from build123d import *

# Parameters (mm, degrees)
BACK_PLATE_DEPTH    = 2
SKETCH3_R           = 39.1
SKETCH3_R_2         = 37.1
BOSS_EXTRUDE2_DEPTH = 4


with BuildPart() as part:
    # Sketch2 → Back Plate (new body)
    with BuildSketch(Plane.XY.offset(1.869079413)):
        with BuildLine():
            ThreePointArc((-22.788405672, 36.551599508), (-51.432945039, 29.694824664), (-43.048816559, 1.45953847))
            ThreePointArc((-43.048816559, 1.45953847), (-43.466528344, 1.037157748), (-43.724007211, 0.501813707))
            ThreePointArc((-43.724007211, 0.501813707), (-43.795371043, 0), (-43.724007211, -0.501813707))
            ThreePointArc((-43.724007211, -0.501813707), (-43.466528344, -1.037157748), (-43.048816559, -1.45953847))
            ThreePointArc((-43.048816559, -1.45953847), (-51.432945039, -29.694824664), (-22.788405672, -36.551599508))
            ThreePointArc((-22.788405672, -36.551599508), (-22.63146913, -37.124538886), (-22.296587024, -37.615194147))
            ThreePointArc((-22.296587024, -37.615194147), (-21.897685521, -37.927903891), (-21.427420187, -38.117007854))
            ThreePointArc((-21.427420187, -38.117007854), (-20.835059214, -38.161696634), (-20.260410887, -38.011137978))
            ThreePointArc((-20.260410887, -38.011137978), (0, -59.389649327), (20.260410887, -38.011137978))
            ThreePointArc((20.260410887, -38.011137978), (20.835059214, -38.161696634), (21.427420187, -38.117007854))
            ThreePointArc((21.427420187, -38.117007854), (21.897685521, -37.927903891), (22.296587024, -37.615194147))
            ThreePointArc((22.296587024, -37.615194147), (22.63146913, -37.124538886), (22.788405672, -36.551599508))
            ThreePointArc((22.788405672, -36.551599508), (51.432945039, -29.694824664), (43.048816559, -1.45953847))
            ThreePointArc((43.048816559, -1.45953847), (43.466528344, -1.037157748), (43.724007211, -0.501813707))
            ThreePointArc((43.724007211, -0.501813707), (43.795371043, 0), (43.724007211, 0.501813707))
            ThreePointArc((43.724007211, 0.501813707), (43.466528344, 1.037157748), (43.048816559, 1.45953847))
            ThreePointArc((43.048816559, 1.45953847), (51.432945039, 29.694824664), (22.788405672, 36.551599508))
            ThreePointArc((22.788405672, 36.551599508), (22.63146913, 37.124538886), (22.296587024, 37.615194147))
            ThreePointArc((22.296587024, 37.615194147), (21.897685521, 37.927903891), (21.427420187, 38.117007854))
            ThreePointArc((21.427420187, 38.117007854), (20.835059214, 38.161696634), (20.260410887, 38.011137978))
            ThreePointArc((20.260410887, 38.011137978), (0, 59.389649327), (-20.260410887, 38.011137978))
            ThreePointArc((-20.260410887, 38.011137978), (-21.897685521, 37.927903891), (-22.788405672, 36.551599508))
        make_face()
        with BuildLine():
            Line((-31, 20.381609357), (-31, -20.381609357))
            ThreePointArc((-31, -20.381609357), (0, -37.1), (31, -20.381609357))
            Line((31, -20.381609357), (31, 20.381609357))
            ThreePointArc((31, 20.381609357), (0, 37.1), (-31, 20.381609357))
        make_face(mode=Mode.SUBTRACT)
    extrude(amount=BACK_PLATE_DEPTH)

    # Sketch3 → Boss-Extrude2 (add)
    with BuildSketch(Plane.XY.offset(3.869079413)):
        Circle(SKETCH3_R)
        with Locations(Location((0, 0, 0), (0, 0, 146.676229541))):
            Circle(SKETCH3_R_2, mode=Mode.SUBTRACT)
    extrude(amount=BOSS_EXTRUDE2_DEPTH)


solid = part.part
Design review of the part built by this model. Coordinates are the model's own, in mm. A direction names the side the tool comes from. Round coordinates to 2 decimals unless told otherwise and drop trailing zeros. Write each loop counter-clockwise with the first axis right and the second up, starting at its lowest first coordinate (ties: lowest second). Pieces come first, ordered by that corner, then holes. Notation, with made-up numbers: (30.25, 10.25) - (83.25, 10.25) arc R23 ccw to (83.25, 33.25) - close; hole circle Ø7 at (52.25, -30). An arc over 180 degrees is marked (long way). Use a Markdown table: item, result. Add a question column.
1. For faces 1 (the face through (33, 0, 3.869)), 2 (the face through (14, -35, 7.869)), list the 3-axis set-ups (+Z, -Z, +X, -X, +Y, -Y) from which the entire face can be reached by the end or side of a thin tool; tool diameter is ignored.
2. Mouldability with a two-part tool opening along Y and no side actions: class faces 3 (the face through (51.2, -30.09, 2.86)), 4 (the face through (-37, 1, 1.869)), 5 (the face through (37.294, 11.745, 5.841)) as +Y half, -Y half, draft (parallel to the pull), parting line (faces both ways), or undercut.
3. Clearance check with flat-ended pins moving along their axes: pin 1 (3 mm diameter, centred on y = 27.5, z = 5, fed in from -X); pin 2 (3 mm diameter, centred on x = -8.5, z = 6, fed in from +Y); pin 3 (1.5 mm diameter, centred on x = -40.5, z = 7, fed in from +Y); pin 4 (1.6 mm diameter, centred on y = 8, z = 3, fed in from -X). State where each tip first meets the part, or that it passes through.
4. We need section C-C (z = 5.2). State the section outline as (x, y) points, then the cut area to 3 significant figures.
5. Wall thickness on probe 1 along Y at (x, z) = (0, 4.9); probe 2 along Y at (x, z) = (46.5, 2.4); probe 3 along Z at (x, y) = (22.5, -32.5): over which ranges is each line inside the solid? List them lowest first.
6. We need section D-D (y = 10.5). State the section outline as (x, z) points.
7. We need section A-A (x = 0). State the section outline as (y, z) points.
8. We need section B-B (y = -12). State the section outline as (x, z) points.
Output:
| question | item | result |
|---|---|---|
| 1 | face 1 | +Z |
| 1 | face 2 | +Z, +X, -X, +Y, -Y |
| 2 | face 3 | undercut |
| 2 | face 4 | draft |
| 2 | face 5 | parting line |
| 3 | pin 1 | stops at x = -52.92 |
| 3 | pin 2 | stops at y = 38.47 |
| 3 | pin 3 | passes through |
| 3 | pin 4 | stops at x = -51.07 |
| 4 | outline | circle Ø78.2 at (0, 0); hole circle Ø74.2 at (0, 0) |
| 4 | area | 479 mm2 |
| 5 | probe 1 | y = -39.1 to -37.1, 37.1 to 39.1 |
| 5 | probe 2 | y = -35.42 to -3.68, 3.68 to 35.42 |
| 5 | probe 3 | z = 1.87 to 3.87 |
| 6 | outline | (-52.02, 1.87) - (-31, 1.87) - (-31, 3.87) - (-35.58, 3.87) - (-35.58, 7.87) - (-37.66, 7.87) - (-37.66, 3.87) - (-52.02, 3.87) - close; (31, 1.87) - (52.02, 1.87) - (52.02, 3.87) - (37.66, 3.87) - (37.66, 7.87) - (35.58, 7.87) - (35.58, 3.87) - (31, 3.87) - close |
| 7 | outline | (-59.39, 1.87) - (-37.1, 1.87) - (-37.1, 7.87) - (-39.1, 7.87) - (-39.1, 3.87) - (-59.39, 3.87) - close; (37.1, 1.87) - (59.39, 1.87) - (59.39, 3.87) - (39.1, 3.87) - (39.1, 7.87) - (37.1, 7.87) - close |
| 8 | outline | (-52.69, 1.87) - (-31, 1.87) - (-31, 3.87) - (-35.11, 3.87) - (-35.11, 7.87) - (-37.21, 7.87) - (-37.21, 3.87) - (-52.69, 3.87) - close; (31, 1.87) - (52.69, 1.87) - (52.69, 3.87) - (37.21, 3.87) - (37.21, 7.87) - (35.11, 7.87) - (35.11, 3.87) - (31, 3.87) - close |
